Source: three-view drawing plus pictorial views. Frame: mm from the lowest corner of the part. Round coordinates to 2 decimals unless told otherwise and drop trailing zeros. Write each loop counter-clockwise with the first axis right and the second up, starting at its lowest first coordinate (ties: lowest second). Pieces come first, ordered by that corner, then holes. Notation, with made-up numbers: M -16.75,48.25 L 25.25,48.25 A15 ccw 25.25,73.25 Z; hole C 77,-12 d8. An arc over 180 degrees is marked long. Answer as CSV lines item,"result". Start each with the question number.
Q1. Section query D-D on z = 14.5. Output: boundary loops of the cut face in (x, y).
Q2. First-contact query: pin 1 (2 mm diameter, centred on x = 26, y = 2.5, fed in from +Z); pin 2 (16 mm diameter, centred on x = 19.05, z = 19.05, fed in from -Y). Flat tips, straight axial feed; report the tip coordinate or a pass-through.
Q3. Section query C-C on x = 65. Output: boundary loops of the cut face in (y, z), and give its area (3 significant figures).
Q4. Ray query, probe 1 along Z at (x, y) = (50.8, 4.75) (1 decimal); probe 2 along Z at (x, y) = (47, 1.75) (1 decimal); probe 3 along X at (y, z) = (4.75, 12.5). Return the intervals inside material, ascending.
Q5. Mould query, pull axis Z, two halves, no side actions, for the marked faces 1 and 2. Classes: pulls with the +Z half, pulls with the -Z half, needs draft (parallel to the pull), parting line crosses it, or undercut.
Q6. Section query B-B on y = 4. Give the number of separate pieces and of enclosed holes in the cut face, and give its area (3 significant figures).
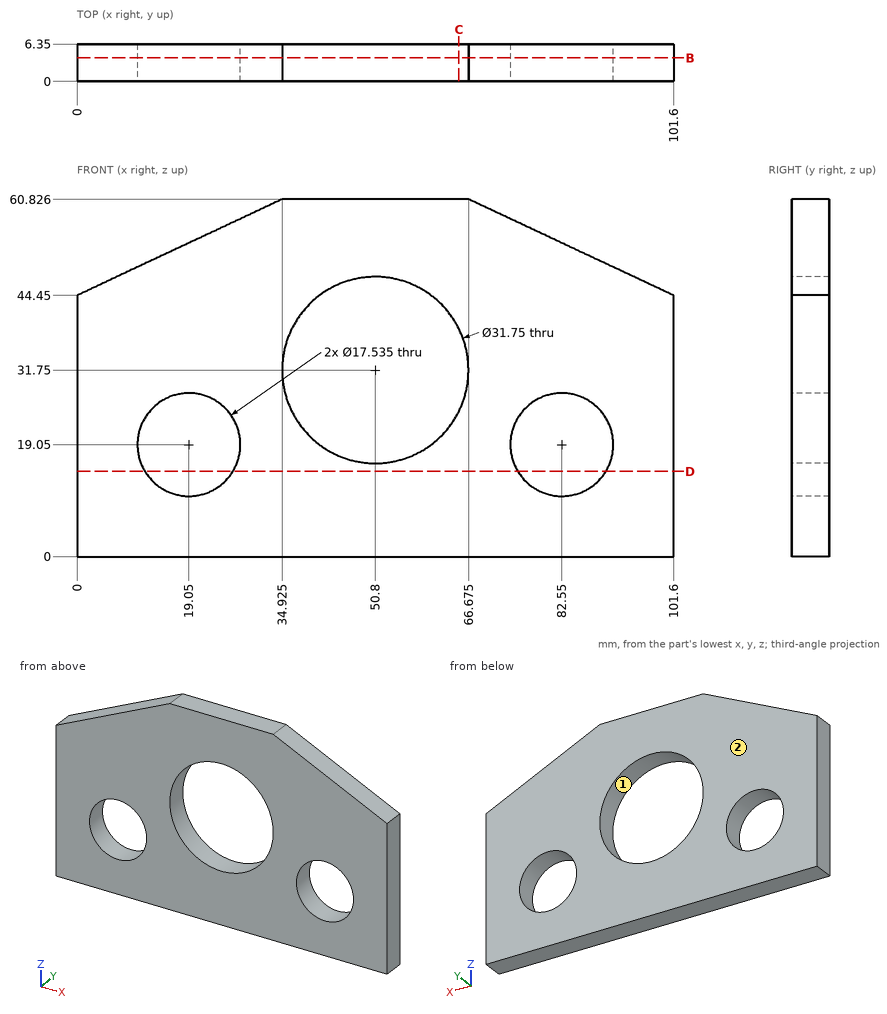
Entries:
1,outline,"M 0,0 L 11.56,0 L 11.56,6.35 L 0,6.35 Z; M 26.54,0 L 75.06,0 L 75.06,6.35 L 26.54,6.35 Z; M 90.04,0 L 101.6,0 L 101.6,6.35 L 90.04,6.35 Z"
2,pin 1,"stops at z = 57.11"
2,pin 2,"passes through"
3,outline,"M 0,0 L 6.35,0 L 6.35,24.65 L 0,24.65 Z; M 0,38.85 L 6.35,38.85 L 6.35,60.83 L 0,60.83 Z"
3,area,"296 mm^2"
4,probe 1,"z = 0 to 15.9, 47.6 to 60.8"
4,probe 2,"z = 0 to 16.3, 47.2 to 60.8"
4,probe 3,"x = 0 to 13.22, 24.88 to 76.72, 88.38 to 101.6"
5,face 1,"undercut"
5,face 2,"needs draft"
6,separate pieces,"1"
6,enclosed holes,"3"
6,area,"4,330 mm^2"
